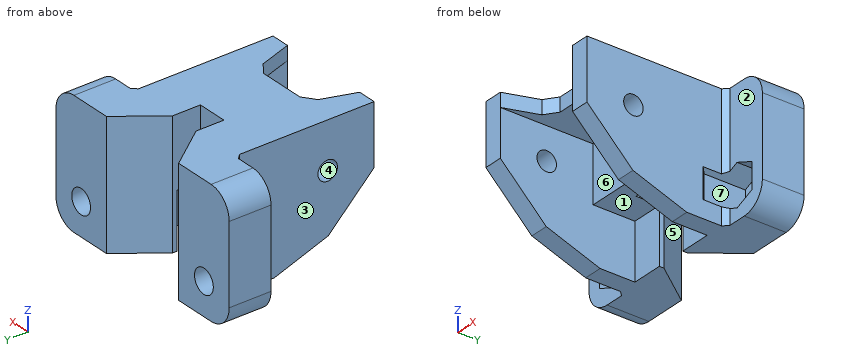
Autodesk Inventor part; units mm, degrees
ref_plane "YZ Plane" through (0, 0, 0) normal (1, 0, 0) x (0, 1, 0)
ref_plane "XZ Plane" through (0, 0, 0) normal (0, 1, 0) x (-1, 0, 0)
ref_plane "XY Plane" through (0, 0, 0) normal (0, 0, 1) x (1, 0, 0)
sketch "Sketch1" plane through (0, 0, 0) normal (0, 0, 1) x (1, 0, 0)
  line L0 (-24, 24) -> (24, 24)
  line L1 (24, 24) -> (24, 15)
  line L2 (24, 15) -> (14, 15)
  line L3 (14, 15) -> (14, -15)
  line L4 (14, -15) -> (10, -15)
  line L5 (10, -15) -> (10, 15)
  line L6 (10, 15) -> (-10, 15)
  line L7 (-10, 15) -> (-10, -15)
  line L8 (-10, -15) -> (-14, -15)
  line L9 (-14, -15) -> (-14, 15)
  line L10 (-14, 15) -> (-24, 15)
  line L11 (-24, 15) -> (-24, 24)
  point P0 (0, 0)
  point P1 (0, 24)
  point P2 (0, 15)
  point P3 (10, 0)
  dimension "d0" = 20
  dimension "d1" = 30
  dimension "d2" = 4
  dimension "d3" = 4
  dimension "d4" = 10
  dimension "d5" = 9
extrude "Extrusion1" add sketch "Sketch1" along normal mid plane 27
sketch "Sketch2" plane through (-24, 24, 13.5) normal (0, 1, 0) x (1, 0, 0)
  circle A0 centre (7, 20) radius 2.6
  circle A1 centre (41, 20) radius 2.6
  line L0 (0, 27) -> (0, 0)
  line L1 (48, 0) -> (48, 27)
  line L2 (0, 27) -> (48, 27)
  point P0 (24, 13.5)
  dimension "d8" = 5.2
  dimension "d9" = 7
  dimension "d10" = 7
  dimension "d52" = 7
extrude "Extrusion2" cut sketch "Sketch2" against normal up to next
sketch "Sketch3" plane through (-24, 15, 13.5) normal (0, -1, 0) x (1, 0, 0)
  circle A0 centre (7, -20) radius 2.6
  circle A1 centre (41, -20) radius 2.6
  line L0 (2.85, -22.76) -> (2.85, -17.24)
  line L1 (2.85, -17.24) -> (7, -15.5)
  line L2 (7, -15.5) -> (11.15, -17.24)
  line L3 (11.15, -17.24) -> (11.15, -22.76)
  line L4 (10, 0) -> (10, -27)
  line L5 (11.15, -22.76) -> (7, -24.5)
  line L6 (7, -24.5) -> (2.85, -22.76)
  point P0 (24, -13.5)
  point P1 (2.85, -20)
  dimension "d13" = 8.3
  dimension "d22" = 9
  dimension "d23" = 8.3
extrude "Extrusion3" cut sketch "Sketch3" against normal blind 5 and the other way blind 4 contours A0 | L0 L1 L2 L4 L5 L6 | L4 L2 L3 L5
mirror "Mirror1" about plane through (0, 0, 0) normal (1, 0, 0) of "Extrusion3"
sketch "Sketch4" plane through (14, -15, 13.5) normal (1, 0, 0) x (0, 0, -1)
  circle A0 centre (10, 10) radius 2.1
  line L0 (0, 0) -> (27, 0)
  point P0 (13.5, 15)
  point P1 (13.5, 0)
  point P2 (13.5, 0)
  dimension "d24" = 4.2
  dimension "d25" = 10
extrude "Extrusion4" cut sketch "Sketch4" against normal up to surface (28 mm away)
fillet "Fillet1" radius 5 4 edges at (-24, 19.5, 13.5) (-24, 19.5, -13.5) (24, 19.5, 13.5) (24, 19.5, -13.5)
chamfer "Chamfer1" distance 1 angle 45 6 edges at (-14, 15, 5.1211) (-14, 11, -6.5) (-14, 15, -11.6211) (14, 15, 5.1211) (14, 11, -6.5) (14, 15, -11.6211)
sketch "Sketch8" plane through (0, 0, 13.5) normal (0, 0, 1) x (1, 0, 0)
  line L0 (-10, 15) -> (10, 15)
  line L1 (10, 15) -> (10, -15)
  line L2 (10, -15) -> (-10, -15)
  line L3 (-10, -15) -> (-10, 15)
  point P0 (0, 0)
extrude "Extrusion7" add sketch "Sketch8" against normal blind 3
sketch "Sketch9" plane through (0, 0, -13.5) normal (0, 0, -1) x (-1, 0, 0)
  line L0 (-10, 5) -> (10, 5)
  line L1 (10, -15) -> (14, -15)
  line L2 (-10, 5) -> (-10, 15)
  line L3 (-10, 15) -> (10, 15)
  line L4 (10, 15) -> (10, 5)
  point P0 (0, 0)
  dimension "d44" = 20
extrude "Extrusion8" add sketch "Sketch9" against normal up to surface (24 mm away)
sketch "Sketch6" plane through (0, 0, 13.5) normal (0, 0, 1) x (1, 0, 0)
  line L0 (-3.25, 15) -> (3.25, 15)
  line L1 (3.25, 15) -> (10, 24)
  line L2 (24, 24) -> (-24, 24)
  line L3 (-3.25, 15) -> (-10, 24)
  line L4 (-10, 24) -> (10, 24)
  line L5 (-14, -15) -> (-10, -15)
  line L6 (-10, 5) -> (10, 5)
  line L7 (-3.25, 15) -> (-3.25, 9)
  line L8 (-3.25, 9) -> (3.25, 9)
  line L9 (3.25, 9) -> (3.25, 15)
  point P0 (0, 0)
  point P1 (0, 15)
  point P2 (0, 24)
  point P3 (-10, 15)
  point P4 (0, 24)
  point P5 (0, 24)
  dimension "d29" = 6.5
  dimension "d30" = 20
  dimension "d47" = 9
  dimension "d48" = 4
extrude "Extrusion5" cut sketch "Sketch6" against normal up to surface (27 mm away)
sketch "Sketch11" plane through (-3.25, 9, 13.5) normal (0, 1, 0) x (1, 0, 0)
  line L0 (13.25, 7.9) -> (13.25, 12.1)
  line L1 (17.25, 12.1) -> (17.25, 7.9)
  circle A0 centre (3.25, 10) radius 2.1
  point P0 (3.25, 13.5)
  point P1 (17.25, 10)
  dimension "d49" = 4.2
extrude "Extrusion9" cut sketch "Sketch11" against normal up to next
sketch "Sketch12" plane through (0, 0, -13.5) normal (0, 0, -1) x (-1, 0, 0)
  line L0 (-10, 5) -> (10, 5)
  line L1 (10, 5) -> (10, 14)
  line L2 (10, 14) -> (-10, 14)
  line L3 (-10, 14) -> (-10, 5)
  point P0 (0, 0)
  point P1 (-10, -15)
  point P2 (10, -15)
  dimension "d53" = 9
extrude "Extrusion10" cut sketch "Sketch12" against normal blind 12
sketch "Sketch13" plane through (14, -15, 13.5) normal (1, 0, 0) x (0, 0, -1)
  line L0 (3, 0) -> (27, 0)
  line L1 (13, 0) -> (27, 14)
  line L2 (27, 29) -> (27, 0)
  line L3 (22.9, 9.9) -> (27, 21.5)
  point P0 (13.5, 15)
  dimension "d58" = 45
  dimension "d59" = 14
  dimension "d62" = 7.5
  dimension "d63" = 4.1
extrude "Extrusion11" cut sketch "Sketch13" against normal through all
sketch "Sketch14" plane through (0, 0, 13.5) normal (0, 0, 1) x (1, 0, 0)
  line L0 (10, -15) -> (7, -6)
  line L1 (7, -6) -> (-7, -6)
  line L2 (-7, -6) -> (-10, -15)
  line L3 (-14, -15) -> (14, -15)
  point P0 (0, 0)
  dimension "d64" = 3
  dimension "d65" = 3
  dimension "d66" = 9
extrude "Extrusion12" cut sketch "Sketch14" against normal up to next
chamfer "Chamfer2" distance 2 angle 45 2 edges at (7, -6, 12) (-7, -6, 12)
equation "\"d3\" = d2"
equation "\"d65\" = d64"
properties part number "holder-GT2-x-carriage-left"
Geometry check sheet. Reference: the model listing, model coordinates, mm. Face numbers are marked on the shaded views. A direction names the side the tool comes from. Coordinates: 2 decimals unless noted, no trailing zeros. Loops run counter-clockwise (first coordinate to the right, second up) from the corner with the lowest first, then second, coordinate; pieces in that order, holes last. Notation, with made-up numbers: (7, 44) - (48, 44) arc R9 cw to (48, 53) - close; hole circle Ø7 at (38, 42). An arc over 180 degrees is marked (long way). One line per item, written item: value. Start each with the question number.
(1) Cross-section at A-A on y = 21. Enter the section's corners in (x, z).
(2) Mould release check, pull along Y, two halves, no side actions. Record for the marked faces 4, 5, 6 and 7: released by +Y, released by -Y, zero draft, split by the parting line, or undercut.
(3) Depth check by flat-ended pin: P1, Ø9, axis at x = 16, z = -6.5, coming from the -Y side; P2, Ø8, axis at y = 4.5, z = -6.5, coming from the +X side; P3, Ø7, axis at y = -7.5, z = 2, coming from the -X side; P4, Ø3, axis at x = -17, z = -7.5, coming from the -Y side. Enter the tip coordinate at first touch or a pass-through.
(4) Cross-section at D-D on y = 7.5. Enter the section's corners in (x, z).
(5) Tool access check on the marked faces 1, 2 and 3. Record the directions out of +Z, -Z, +X, -X, +Y, -Y that give a thin tool (end or side, any length) a straight path to the whole face; none if there is none.
(6) Material ranges on line 1 (X direction, y = 14, z = 3.25); line 2 (Y direction, x = -11.3, z = 3.5); line 3 (Z direction, x = 17, y = 22.5), recorded low to high. Write a range as [from, to].
(7) Cross-section at C-C on x = 0. Enter the section's corners in (y, z), plus the area to 3 significant figures.
(8) Cross-section at B-B on z = 3.5. Count the separate pieces of the cut face and the enclosed holes in it, plus the area to 3 significant figures.
Results below:
1. outline: (-24, -8.5) arc R5 ccw to (-19, -13.5) - (-7.75, -13.5) - (-7.75, 13.5) - (-19, 13.5) arc R5 ccw to (-24, 8.5) - close; (7.75, -13.5) - (19, -13.5) arc R5 ccw to (24, -8.5) - (24, 8.5) arc R5 ccw to (19, 13.5) - (7.75, 13.5) - close; hole circle Ø5.2 at (-17, -6.5); hole circle Ø5.2 at (17, -6.5)
2. face 4: undercut
2. face 5: released by +Y
2. face 6: released by -Y
2. face 7: undercut
3. P1: stops at y = -12.03
3. P2: stops at x = 14
3. P3: stops at x = -14
3. P4: passes through
4. outline: (-14, -13.5) - (-10, -13.5) - (-10, -1.5) - (10, -1.5) - (10, -13.5) - (14, -13.5) - (14, 13.5) - (-14, 13.5) - close; hole circle Ø4.2 at (0, 3.5)
5. face 1: -Z, -Y
5. face 2: +Z, -Z, +X, -Y
5. face 3: +Z, -Z, -X, -Y
6. line 1: x = [-14, -3.25], [3.25, 14]
6. line 2: y = [-15, -7.1], [-2.9, 24]
6. line 3: z = [-13.5, -9.1], [-3.9, 13.5]
7. outline: (-6, 10.5) - (5, 10.5) - (5, 5.6) - (9, 5.6) - (9, 13.5) - (-6, 13.5) - close; (5, -1.5) - (9, -1.5) - (9, 1.4) - (5, 1.4) - close
7. area: 76.2 mm2
8. separate pieces: 4
8. enclosed holes: 0
8. area: 664 mm2
